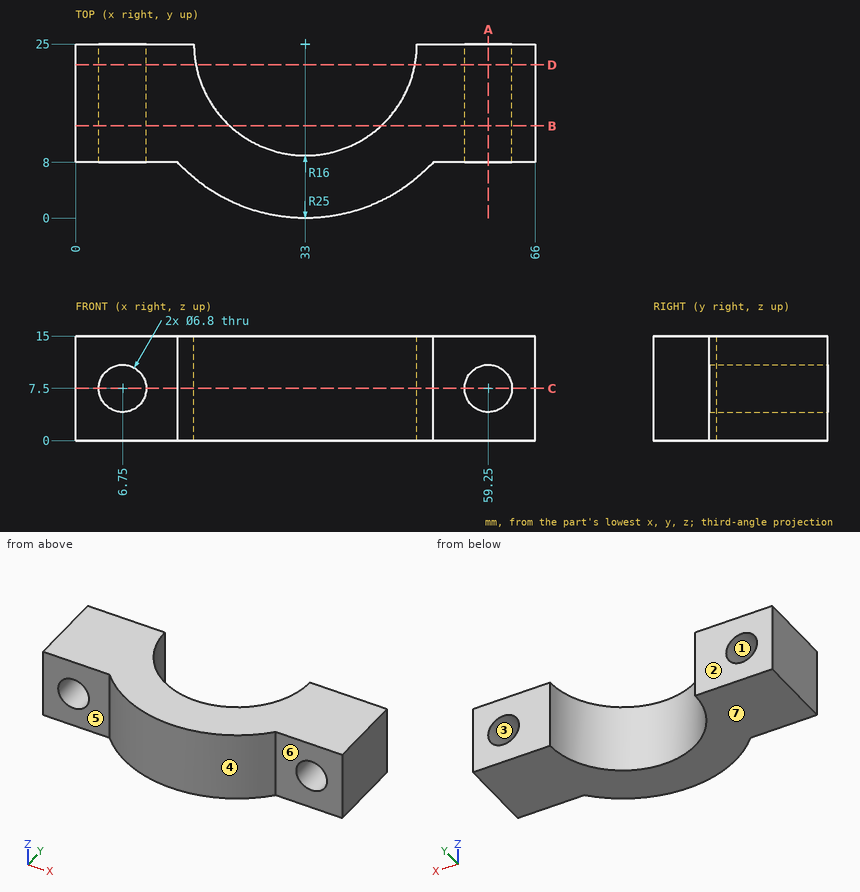
Verification items for this drawing (mm, ordinates from the low corner). A direction names the side the tool comes from. Coordinates: 2 decimals unless noted, no trailing zeros. Loops run counter-clockwise (first coordinate to the right, second up) from the corner with the lowest first, then second, coordinate; pieces in that order, holes last.
Item 1: Access from +Z, -Z, +X, -X, +Y, -Y to the whole of each face (thin tool, end or side, straight path). Record for the marked faces 5, 6 and 7.
Item 2: Thickness scan on line 1 (Z direction, x = 59.25, y = 17.5); line 2 (X direction, y = 20.75, z = 8.75); line 3 (Y direction, x = 11.5, z = 1.5). Record the ranges inside material, lowest first.
Item 3: Sectioned sample at C-C, the plane z = 7.5. Record the boundary of the cut face in (x, y), then the cut area to 3 significant figures.
Item 4: Go/stop test with flat-tipped pins: pin 1 Ø4 at (y, z) = (13, 3) entering from -X; pin 2 Ø2 at (x, z) = (33.5, 5.5) entering from +Y; pin 3 Ø3 at (y, z) = (4.5, 9.5) entering from +X; pin 4 Ø4.5 at (x, z) = (58, 4.5) entering from -Y. Record where each tip stops, or that it passes through.
Item 5: Sectioned sample at B-B, the plane y = 13.25. Record the boundary of the cut face in (x, z).
Item 6: Release check for a two-part mould opening along X. For the marked faces 1, 2, 3 and 4 record: released by +X, released by -X, zero draft, split by the parting line, or undercut.
Item 7: Sectioned sample at D-D, the plane y = 22. Record the boundary of the cut face in (x, z), then the cut area to 3 significant figures.
Item 8: Sectioned sample at A-A, the plane x = 59.25. Record the boundary of the cut face in (y, z).
Check result:
1. face 5: +Z, -Z, -X, -Y
1. face 6: +Z, -Z, +X, -Y
1. face 7: -Z, +X, -X, +Y, -Y
2. line 1: z = 0 to 4.1, 10.9 to 15
2. line 2: x = 0 to 3.59, 9.91 to 17.57, 48.43 to 56.09, 62.41 to 66
2. line 3: y = 8 to 25
3. outline: (0, 8) - (3.35, 8) - (3.35, 25) - (0, 25) - close; (10.15, 8) - (14.67, 8) arc R25 ccw to (51.33, 8) - (55.85, 8) - (55.85, 25) - (49, 25) arc R16 cw to (17, 25) - (10.15, 25) - close; (62.65, 8) - (66, 8) - (66, 25) - (62.65, 25) - close
3. area: 691 mm2
4. pin 1: stops at x = 0
4. pin 2: stops at y = 9.07
4. pin 3: stops at x = 49.25
4. pin 4: stops at y = 8
5. outline: (0, 0) - (22.14, 0) - (22.14, 15) - (0, 15) - close; (43.86, 0) - (66, 0) - (66, 15) - (43.86, 15) - close; hole circle Ø6.8 at (6.75, 7.5); hole circle Ø6.8 at (59.25, 7.5)
6. face 1: undercut
6. face 2: zero draft
6. face 3: undercut
6. face 4: split by the parting line
7. outline: (0, 0) - (17.28, 0) - (17.28, 15) - (0, 15) - close; (48.72, 0) - (66, 0) - (66, 15) - (48.72, 15) - close; hole circle Ø6.8 at (6.75, 7.5); hole circle Ø6.8 at (59.25, 7.5)
7. area: 446 mm2
8. outline: (8, 0) - (25, 0) - (25, 4.1) - (8, 4.1) - close; (8, 10.9) - (25, 10.9) - (25, 15) - (8, 15) - close
